```python
from build123d import *

# Parameters (mm, degrees)
SKETCH1_W           = 6.096
SKETCH1_H           = 13.208
BOSS_EXTRUDE1_DEPTH = 114.3
SKETCH3_W           = 131.064
SKETCH3_H           = 55.245
SKETCH3_H_2         = 51.435
CUT_EXTRUDE2_DEPTH  = 304.8
BOSS_EXTRUDE2_DEPTH = 114.3


with BuildPart() as part:
    # Sketch1 → Boss-Extrude1 (new body)
    with BuildSketch(Plane(origin=(0, 0, 0), x_dir=(1, 0, 0), z_dir=(0, 1, 0))):
        Polygon((72.644, 78.486), (0, 78.486), (0, 0), (72.644, 0), (72.644, 56.572009751), (72.644, 65.278), align=None)
        with Locations((75.692, 71.882)):
            Rectangle(SKETCH1_W, SKETCH1_H)
        Polygon((72.644, 0), (0, 0), (0, -78.486), (72.644, -78.486), (72.644, -65.278), (72.644, -56.572009751), align=None)
        Polygon((0, -78.486), (0, 0), (-72.644, 0), (-72.644, -56.572009751), (-72.644, -65.278), (-72.644, -78.486), align=None)
        with Locations((-75.692, -71.882)):
            Rectangle(SKETCH1_W, SKETCH1_H)
        Polygon((0, 0), (0, 78.486), (-72.644, 78.486), (-72.644, 65.278), (-72.644, 56.572009751), (-72.644, 0), align=None)
        with Locations((-75.692, 71.882)):
            Rectangle(SKETCH1_W, SKETCH1_H)
        with Locations((75.692, -71.882)):
            Rectangle(SKETCH1_W, SKETCH1_H)
    extrude(amount=BOSS_EXTRUDE1_DEPTH)

    # Sketch3 → Cut-Extrude2 (cut)
    with BuildSketch(Plane.XY.offset(78.486)):
        with Locations((0, 31.4325)):
            Rectangle(SKETCH3_W, SKETCH3_H)
        with Locations((0, 88.5825)):
            Rectangle(SKETCH3_W, SKETCH3_H_2)
    extrude(amount=-CUT_EXTRUDE2_DEPTH, mode=Mode.SUBTRACT)

    # Sketch4 → Boss-Extrude2 (add)
    with BuildSketch(Plane.XZ):
        Polygon((-78.74, 65.278), (-72.644, 65.278), (-72.644, 56.572009751), align=None)
        Polygon((-72.644, -65.278), (-78.74, -65.278), (-72.644, -56.572009751), align=None)
        Polygon((72.644, -65.278), (72.644, -56.572009751), (78.74, -65.278), align=None)
        Polygon((72.644, 56.572009751), (72.644, 65.278), (78.74, 65.278), align=None)
    extrude(amount=-BOSS_EXTRUDE2_DEPTH)


solid = part.part
```
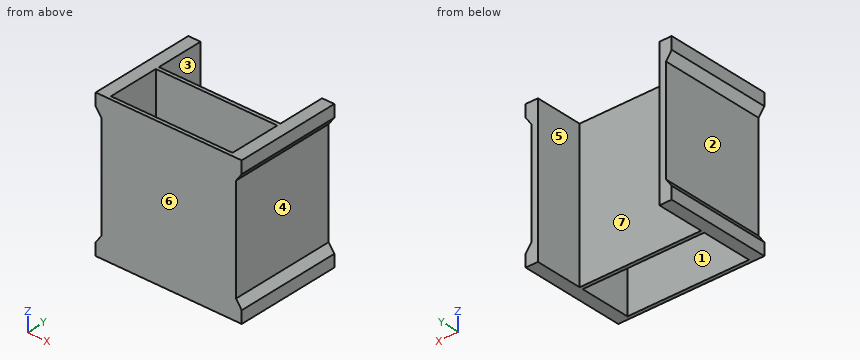
Read the model definition and answer for the solid it produces. Units are mm, in the model's axes. Face numbers are marked on the shaded views. A direction names the side the tool comes from. Round coordinates to 2 decimals unless told otherwise and drop trailing zeros. Write each loop counter-clockwise with the first axis right and the second up, starting at its lowest first coordinate (ties: lowest second). Pieces come first, ordered by that corner, then holes. Notation, with made-up numbers: (-38, -17) -> (-18, -17) arc R26 ccw to (-18, -1) -> close; hole circle Ø9 at (23.5, -20). An arc over 180 degrees is marked (long way). Answer in a Markdown table with one row per item. Add a question column.
1) Consider line 1 (X direction, y = 63, z = -24); line 2 (Y direction, x = 51.5, z = -62.5) (3 decimals); line 3 (X direction, y = 48, z = -61.5). Determine where each line is inside the solid, lowest interval first.
2) Find section D-D, the plane z = -61. Determine the outline of the cut face in (x, y) (3 decimals), and give its area (3 significant figures).
3) Find section A-A, the plane y = 69.5. Determine the outline of the cut face in (x, z), and give its area (3 significant figures).
4) Given P1, Ø1, axis at y = 70.5, z = -55.5, coming from the +X side; P2, Ø10, axis at x = -31.5, z = 56.5, coming from the +Y side (3 decimals); P3, Ø10, axis at y = 29.5, z = 25.5, coming from the -X side, each flat-ended and moving along its own axis, determine where each tip first touches the part or whether it passes through.
5) Which of the six approach directions +Z, -Z, +X, -X, +Y, -Y give full straight-line access (tool end or side, diameter ignored) to the marked faces 1, 2 and 3?
6) Determine the mould class of the marked faces 4, 5, 6 and 7 for opening direction X: pulls with the +X half, pulls with the -X half, needs draft (parallel to the pull), parting line crosses it, or undercut.
7) Find section B-B, the plane x = 28. Determine the outline of the cut face in (y, z) (3 decimals).
8) Find section C-C, the plane z = 47.5. Determine the outline of the cut face in (x, y) (3 decimals), and give its area (3 significant figures).
Findings below:
| question | item | result |
|---|---|---|
| 1 | line 1 | -72.64 to -65.53, 65.53 to 72.64 |
| 1 | line 2 | 0 to 3.81, 59.055 to 62.865 |
| 1 | line 3 | -76.09 to -65.53, 65.53 to 76.09 |
| 2 | outline | (-75.745, 0) -> (75.745, 0) -> (75.745, 114.3) -> (65.532, 114.3) -> (65.532, 62.865) -> (-65.532, 62.865) -> (-65.532, 114.3) -> (-75.745, 114.3) -> close; hole (-65.532, 3.81) -> (65.532, 3.81) -> (65.532, 59.055) -> (-65.532, 59.055) -> close |
| 2 | area | 3,330 mm² |
| 3 | outline | (-78.74, -78.49) -> (-65.53, -78.49) -> (-65.53, 78.49) -> (-78.74, 78.49) -> (-78.74, 65.28) -> (-72.64, 56.57) -> (-72.64, -56.57) -> (-78.74, -65.28) -> close; (65.53, -78.49) -> (78.74, -78.49) -> (78.74, -65.28) -> (72.64, -56.57) -> (72.64, 56.57) -> (78.74, 65.28) -> (78.74, 78.49) -> (65.53, 78.49) -> close |
| 3 | area | 2,660 mm² |
| 4 | P1 | x = 72.64 |
| 4 | P2 | y = 62.865 |
| 4 | P3 | x = -72.64 |
| 5 | face 1 | +Z, -Z |
| 5 | face 2 | -X, +Y, -Y |
| 5 | face 3 | +Z, -Z, +Y |
| 6 | face 4 | pulls with the +X half |
| 6 | face 5 | undercut |
| 6 | face 6 | needs draft |
| 6 | face 7 | undercut |
| 7 | outline | (0, -78.486) -> (3.81, -78.486) -> (3.81, 78.486) -> (0, 78.486) -> close; (59.055, -78.486) -> (62.865, -78.486) -> (62.865, 78.486) -> (59.055, 78.486) -> close |
| 8 | outline | (-72.644, 0) -> (72.644, 0) -> (72.644, 114.3) -> (65.532, 114.3) -> (65.532, 62.865) -> (-65.532, 62.865) -> (-65.532, 114.3) -> (-72.644, 114.3) -> close; hole (-65.532, 3.81) -> (65.532, 3.81) -> (65.532, 59.055) -> (-65.532, 59.055) -> close |
| 8 | area | 2,620 mm² |
